Work out the finished part from the listing and answer in its coordinate system (mm). A direction names the side the tool comes from. Coordinates: 2 decimals unless noted, no trailing zeros. Order: outer loops, then holes, each group sorted by start corner. A loop starts at its lowest first (then second) coordinate and runs counter-clockwise, first axis right, second up. Notation, with made-up numbers: M 11.25,62.5 L 32.25,62.5 A32 ccw 32.25,92.5 Z; hole C 78.25,79.25 d5. An arc over 180 degrees is marked long. Use a Markdown table: item, result.
from build123d import *

# Parameters (mm, degrees)
SKETCH1_R                  = 6.3
BOSS_EXTRUDE1_DEPTH        = 25
F_8_0_199_DIAMETER_HOLE1_D = 5.0546
CUT_EXTRUDE2_START         = -3
SKETCH5_R                  = 5.08
CUT_EXTRUDE2_DEPTH         = 36.191785898
SKETCH6_W                  = 2
SKETCH6_H                  = 2
BOSS_EXTRUDE2_DEPTH        = 25
FILLET1_R                  = 1


with BuildPart() as part:
    # Sketch1 → Boss-Extrude1 (new body)
    with BuildSketch(Plane.XY):
        with BuildLine():
            Line((14.7, 8.3), (14.7, 15.55))
            Line((14.7, 15.55), (-14.7, 15.55))
            Line((-14.7, 15.55), (-14.7, 8.3))
            Line((-14.7, 8.3), (-8.277443092, -4.239567886))
            ThreePointArc((-8.277443092, -4.239567886), (-0.883815497, -9.25790852), (7.325770018, -5.729144233))
            Line((7.325770018, -5.729144233), (14.7, 8.3))
        make_face()
        Circle(SKETCH1_R, mode=Mode.SUBTRACT)
    extrude(amount=BOSS_EXTRUDE1_DEPTH)

    # #8 (0.199) Diameter Hole1 (through all)
    with Locations(Plane(origin=(0, 15.55, 0), x_dir=(1, 0, 0), z_dir=(0, 1, 0))):
        with Locations((0, -12.5)):
            Hole(F_8_0_199_DIAMETER_HOLE1_D / 2)

    # Sketch5 → Cut-Extrude2 (cut, through all)
    with BuildSketch(Plane(origin=(0, 15.55, 0), x_dir=(1, 0, 0), z_dir=(0, 1, 0)).offset(CUT_EXTRUDE2_START)):
        with Locations(Location((0, -12.5, 0), (0, 0, 180))):
            Circle(SKETCH5_R)
    extrude(amount=-CUT_EXTRUDE2_DEPTH, mode=Mode.SUBTRACT)

    # Sketch6 → Boss-Extrude2 (add)
    with BuildSketch(Plane(origin=(0, 0, 0), x_dir=(-1, 0, 0), z_dir=(0, 0, -1))):
        with Locations((13.7, 16.55)):
            Rectangle(SKETCH6_W, SKETCH6_H)
        with Locations((-13.7, 16.55)):
            Rectangle(SKETCH6_W, SKETCH6_H)
    extrude(amount=-BOSS_EXTRUDE2_DEPTH)

    # Fillet1
    fillet1_edges = [part.edges().sort_by_distance(p)[0] for p in [
        (-14.7, 8.3, 12.5),
        (14.7, 8.3, 12.5),
        (-12.7, 17.55, 12.5),
        (12.7, 17.55, 12.5),
    ]]
    fillet(fillet1_edges, radius=FILLET1_R)


solid = part.part
1. Section B-B on y = 0 is taken. Determine the outline of the cut face in (x, z), then the cut area to 3 significant figures.
Answers below:
| item | result |
|---|---|
| outline | M -10.45,0 L -6.3,0 L -6.3,25 L -10.45,25 Z; M 6.3,0 L 10.34,0 L 10.34,25 L 6.3,25 Z |
| area | 205 mm² |
2. For faces 1 (the face through (12.7, 16, 12)), 2 (the face through (14, 17.55, 12)), 3 (the face through (-2.34, 9.18, 7.99)), determine the directions among +Z, -Z, +X, -X, +Y, -Y from which every point of the face is accessible in a straight line to the end or side of a thin tool.
Answers below:
| item | result |
|---|---|
| face 1 | +Z, -Z, +Y |
| face 2 | +Z, -Z, +X, -X, +Y |
| face 3 | -Y |
3. Section C-C on z = 22 is taken. Determine the outline of the cut face in (x, y), then the cut area to 3 significant figures.
Answers below:
| item | result |
|---|---|
| outline | M -14.7,8.54 A1 ccw -14.59,8.09 L -8.28,-4.24 A9.3 ccw 7.33,-5.73 L 14.59,8.08 A1 ccw 14.7,8.55 L 14.7,17.55 L 13.7,17.55 A1 ccw 12.7,16.55 L 12.7,15.55 L -12.7,15.55 L -12.7,16.55 A1 ccw -13.7,17.55 L -14.7,17.55 Z; hole C 0,0 d12.6 |
| area | 443 mm² |
4. Section D-D on x = 4 is taken. Determine the outline of the cut face in (y, z), then the cut area to 3 significant figures.
Answers below:
| item | result |
|---|---|
| outline | M -8.4,0 L -4.87,0 L -4.87,9.37 L -8.4,9.37 Z; M -8.4,15.63 L -4.87,15.63 L -4.87,25 L -8.4,25 Z; M 4.87,0 L 15.55,0 L 15.55,25 L 4.87,25 L 4.87,15.63 L 12.55,15.63 L 12.55,9.37 L 4.87,9.37 Z |
| area | 285 mm² |
5. Flat-ended cylindrical pins translate along their axes: P1, Ø5, axis at x = 10.5, y = 3, coming from the -Z side; P2, Ø3, axis at x = 0.5, z = 11.5, coming from the -Y side; P3, Ø8, axis at x = -8.5, z = 6, coming from the +Y side; P4, Ø2, axis at x = -11, z = 18.5, coming from the -Y side. Find the tip coordinate at first contact, or state that the pin passes through.
Answers below:
| item | result |
|---|---|
| P1 | z = 0 |
| P2 | y = 12.55 |
| P3 | y = 15.55 |
| P4 | y = -0.88 |
6. For a pull along X with two mould halves and no side action, classify faces 4 (the face through (0, 7, 0)), 5 (the face through (14.7, 13, 12)), 6 (the face through (4.03, -7.1, 9.41)) as +X half, -X half, draft (parallel to the pull), parting line (faces both ways), or undercut.
Answers below:
| item | result |
|---|---|
| face 4 | draft |
| face 5 | +X half |
| face 6 | undercut |
7. Section A-A on x = 0 is taken. Determine the outline of the cut face in (y, z).
Answers below:
| item | result |
|---|---|
| outline | M -9.3,0 L -6.3,0 L -6.3,7.42 L -9.3,7.42 Z; M -9.3,17.58 L -6.3,17.58 L -6.3,25 L -9.3,25 Z; M 6.3,0 L 15.55,0 L 15.55,9.97 L 12.55,9.97 L 12.55,7.42 L 6.3,7.42 Z; M 6.3,17.58 L 12.55,17.58 L 12.55,15.03 L 15.55,15.03 L 15.55,25 L 6.3,25 Z |
8. Find the intervals of material crossed by probe 1 along X at (y, z) = (14.65, 12.5); probe 2 along X at (y, z) = (15.75, 16.5); probe 3 along Z at (x, y) = (0, 7.75), in increasing order.
Answers below:
| item | result |
|---|---|
| probe 1 | -14.7 to -2.53, 2.53 to 14.7 |
| probe 2 | -14.7 to -12.7, 12.7 to 14.7 |
| probe 3 | 0 to 7.42, 17.58 to 25 |
